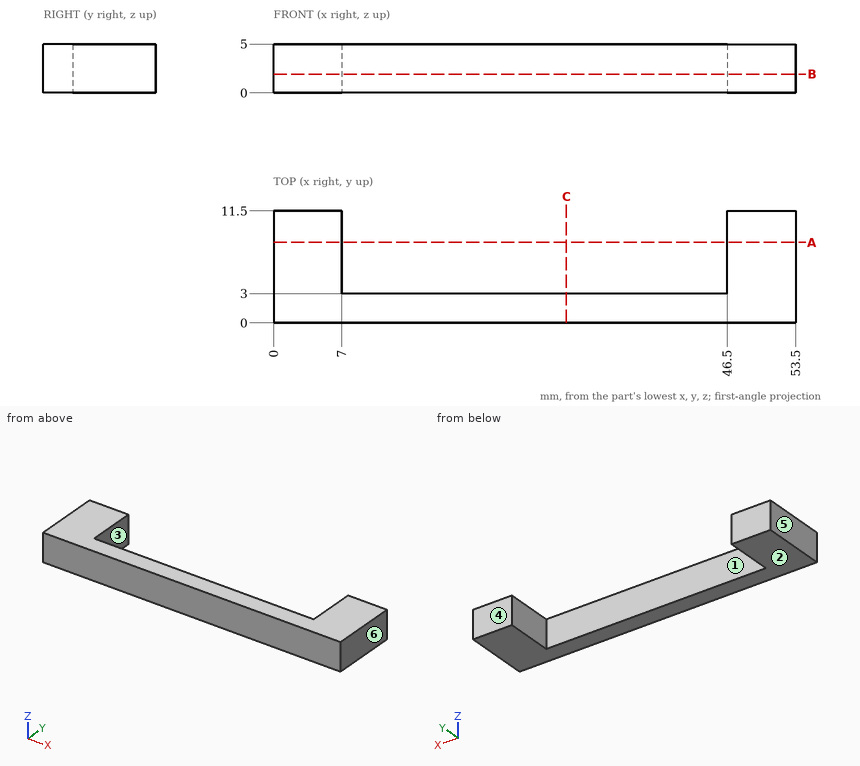
The figure shows three views and two pictorial views of one solid part (mm, origin at its lowest corner). Answer the questions. A direction names the side the tool comes from. Give positions to 0.01 mm unless a question says otherwise; leave off trailing zeros. Loops run counter-clockwise (first coordinate to the right, second up) from the corner with the lowest first, then second, coordinate; pieces in that order, holes last. Notation, with made-up numbers: (88.25, 57.5) - (127.25, 57.5) arc R24 ccw to (127.25, 71.5) - close; hole circle Ø2 at (-34.5, 84). An arc over 180 degrees is marked (long way). Use one line per item in the form item = value.
1. Section B-B on z = 1.9 is taken. Give the vertices of the cut face in (x, y).
Calculated:
outline = (0, 0) - (53.5, 0) - (53.5, 11.5) - (46.5, 11.5) - (46.5, 3) - (7, 3) - (7, 11.5) - (0, 11.5) - close
2. Given pin 1 Ø1.5 at (x, z) = (23.5, 3) entering from +Y, flat-ended and moving along its own axis, determine where the tip first touches the part or whether it passes through.
Calculated:
pin_1 = 3
3. Section A-A on y = 8.25 is taken. Give the vertices of the cut face in (x, z).
Calculated:
outline = (0, 0) - (7, 0) - (7, 5) - (0, 5) - close; (46.5, 0) - (53.5, 0) - (53.5, 5) - (46.5, 5) - close
4. The mould has two halves that part along X. Classify the marked faces 3, 4, 5 and 6: pulls with the +X half, pulls with the -X half, needs draft (parallel to the pull), parting line crosses it, or undercut.
Calculated:
face_3 = undercut
face_4 = needs draft
face_5 = pulls with the -X half
face_6 = pulls with the +X half
5. Section C-C on x = 30 is taken. Give the vertices of the cut face in (y, z).
Calculated:
outline = (0, 0) - (3, 0) - (3, 5) - (0, 5) - close
6. Which of the six approach directions +Z, -Z, +X, -X, +Y, -Y give full straight-line access (tool end or side, diameter ignored) to the marked faces 1 and 2?
Calculated:
face_1 = +Z, -Z, +Y
face_2 = -Z, +X, -X, +Y, -Y
7. Find the intervals of material crossed by line 1 along X through (y, z) = (9, 1.95); line 2 along Y through (x, z) = (18.5, 1.05), in increasing order. Write a range as [from, to].
Calculated:
line_1 = [0, 7], [46.5, 53.5]
line_2 = [0, 3]
